```python
from build123d import *

# Parameters (mm, degrees)
PAD_DEPTH    = 20
FILLET_R     = 8
THICKNESS_T  = -1.5
SKETCH001_W  = 1.5
SKETCH001_H  = 20
PAD001_DEPTH = 5


with BuildPart() as part:
    # Sketch → Pad (new body)
    with BuildSketch(Plane.XY):
        Polygon((0, 0), (18, 0), (18, -8), (-4.208438, -11.5), (-12.5, -8), (0, -3), align=None)
    extrude(amount=PAD_DEPTH)

    # Fillet
    fillet_edges = [part.edges().sort_by_distance(p)[0] for p in [
        (18, -8, 10),
    ]]
    fillet(fillet_edges, radius=FILLET_R)

    # Thickness
    thickness_openings = [part.faces().sort_by_distance(p)[0] for p in [
        (9, 0, 10),
        (-8.354219, -9.75, 10),
    ]]
    offset(amount=THICKNESS_T, openings=thickness_openings)

    # Sketch001 → Pad001 (new body)
    with BuildSketch(Plane(origin=(0, 0, 0), x_dir=(-1, 0, 0), z_dir=(0, 1, 0))):
        with Locations((-17.25, 10)):
            Rectangle(SKETCH001_W, SKETCH001_H)
        with Locations((-0.75, 10)):
            Rectangle(SKETCH001_W, SKETCH001_H)
    extrude(amount=PAD001_DEPTH)


solid = part.part
```
Verification items for the finished model (mm, model axes). A direction names the side the tool comes from. Round coordinates to 2 decimals unless told otherwise and drop trailing zeros. Order: outer loops, then holes, each group sorted by start corner. A loop starts at its lowest first (then second) coordinate and runs counter-clockwise, first axis right, second up. Notation, with made-up numbers: (10, -10) - (68, -10) arc R28 cw to (68, 11) - close; hole circle Ø9 at (-11.75, -39). An arc over 180 degrees is marked (long way). Use CSV: the item, a comma, the result in double quotes.
(1) Section check A-A on z = 12.25. Record the boundary of the cut face in (x, y).
Entries:
outline,"(-12.5, -8) - (-10.53, -8.83) - (0.56, -4.39) arc R1.5 ccw to (1.5, -3) - (1.5, 5) - (0, 5) - (0, -3) - close; (-6.83, -10.39) - (-4.21, -11.5) - (11.25, -9.06) arc R8 ccw to (18, -1.16) - (18, 5) - (16.5, 5) - (16.5, -1.16) arc R6.5 cw to (11.01, -7.58) - close"
(2) Section check D-D on y = -5.5. Record the boundary of the cut face in (x, z).
Entries:
outline,"(-6.25, 0) - (16.72, 0) - (16.72, 20) - (-6.25, 20) - close; hole (-2.21, 1.5) - (14.84, 1.5) - (14.84, 18.5) - (-2.21, 18.5) - close"
(3) Section check B-B on y = 4. Record the boundary of the cut face in (x, z), and give its area (3 significant figures).
Entries:
outline,"(0, 0) - (1.5, 0) - (1.5, 20) - (0, 20) - close; (16.5, 0) - (18, 0) - (18, 20) - (16.5, 20) - close"
area,"60.0 mm^2"
(4) Gauge pin test, flat ends, axial feed: pin 1 Ø1.6 at (x, z) = (8, 19) entering from +Y; pin 2 Ø1.5 at (y, z) = (0, 17.5) entering from -X; pin 3 Ø2 at (x, z) = (-4.5, 9) entering from -Y. Record the tip position at first contact, or that the pin passes through.
Entries:
pin 1,"y = 0"
pin 2,"x = 0"
pin 3,"y = -11.5"
(5) Section check C-C on x = 1. Record the boundary of the cut face in (y, z).
Entries:
outline,"(-10.68, 0) - (5, 0) - (5, 20) - (-10.68, 20) - close; hole (-9.16, 1.5) - (-4.12, 1.5) - (-4.12, 18.5) - (-9.16, 18.5) - close"
(6) Thickness scan on probe 1 along Z at (x, y) = (-6.5, -9.5); probe 2 along X at (y, z) = (1.5, 1); probe 3 along Y at (x, z) = (-0.5, 11). Record the ranges inside material, lowest first. Write a range as from..to.
Entries:
probe 1,"0..1.5, 18.5..20"
probe 2,"0..1.5, 16.5..18"
probe 3,"-10.92..-9.4, -4.82..-3.2"
(7) Access from +Z, -Z, +X, -X, +Y, -Y to the whole of each face (thin tool, end or side, straight path). Record for faces 1 (the face through (2.22, -8.97, 9.88)), 2 (the face through (0, 1, 10)), 3 (the face through (9, 0, 1)).
Entries:
face 1,"none"
face 2,"+Z, -Z, -X, +Y"
face 3,"+Z, -Z, +Y"
(8) Mould release check, pull along X, two halves, no side actions. Record for faces 4 (the face through (16.13, -6.3, 10.14)), 5 (the face through (1, 5, 10)), 6 (the face through (1.5, 1, 10)): released by +X, released by -X, zero draft, split by the parting line, or undercut.
Entries:
face 4,"released by +X"
face 5,"zero draft"
face 6,"undercut"
